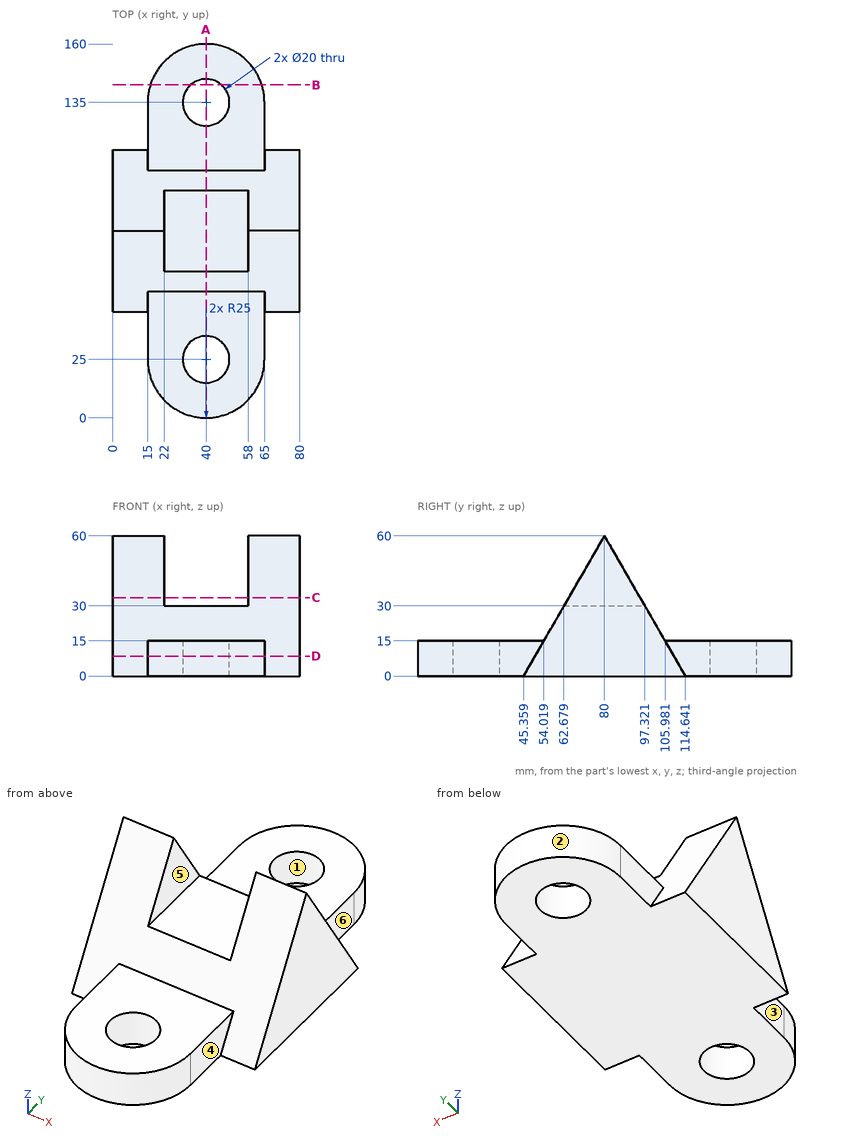
Study the drawing (mm; zero at the part's minimum x, y, z) and answer. A direction names the side the tool comes from. Round coordinates to 2 decimals unless told otherwise and drop trailing zeros. Write each loop counter-clockwise with the first axis right and the second up, starting at its lowest first coordinate (ties: lowest second). Pieces come first, ordered by that corner, then holes. Notation, with made-up numbers: (77.5, -40) - (110.5, -40) arc R13 cw to (110.5, -21) - close; hole circle Ø3 at (-10.5, 54.25). An arc over 180 degrees is marked (long way). Use a Markdown table: item, result. Add a question column.
1. For a pull along Y with two mould halves and no side action, classify the marked faces 1, 2 and 3 as +Y half, -Y half, draft (parallel to the pull), parting line (faces both ways), or undercut.
2. The part is cut by section C-C (z = 33.5). Write down the section's boundary in (x, y).
3. Consider line 1 (Y direction, x = 40, z = 5.5); line 2 (Z direction, x = 59, y = 121.5); line 3 (X direction, y = 126, z = 11) (1 decimal). Determine where each line is inside the solid, lowest interval first.
4. Flat-ended cylindrical pins translate along their axes: P1, Ø4.5, axis at y = 41, z = 5.5, coming from the -X side; P2, Ø6, axis at x = 57, z = 18.5, coming from the +Y side; P3, Ø1.5, axis at x = 26, z = 24, coming from the -Y side. Find the tip coordinate at first contact, or state that the pin passes through.
5. The part is cut by section B-B (y = 142.5). Write down the section's boundary in (x, z) (1 decimal), and give its area (3 significant figures).
6. The part is cut by section D-D (z = 8.5). Write down the section's boundary in (x, y), and give its area (3 significant figures).
7. The part is cut by section A-A (x = 40). Write down the section's boundary in (y, z).
8. A tool of negligible diameter and unlimited length cuts with its end or side. For the marked faces 4, 5 and 6, from which of +Z, -Z, +X, -X, +Y, -Y can it reach the whole face along a straight path? Write none if from no direction.
Reported:
| question | item | result |
|---|---|---|
| 1 | face 1 | undercut |
| 1 | face 2 | +Y half |
| 1 | face 3 | draft |
| 2 | outline | (0, 64.7) - (22, 64.7) - (22, 95.3) - (0, 95.3) - close; (58, 64.7) - (80, 64.7) - (80, 95.3) - (58, 95.3) - close |
| 3 | line 1 | 0 to 15, 35 to 125, 145 to 160 |
| 3 | line 2 | 0 to 15 |
| 3 | line 3 | 15 to 35.6, 44.4 to 65 |
| 4 | P1 | x = 15 |
| 4 | P2 | y = 105.69 |
| 4 | P3 | y = 58.78 |
| 5 | outline | (16.2, 0) - (33.4, 0) - (33.4, 15) - (16.2, 15) - close; (46.6, 0) - (63.8, 0) - (63.8, 15) - (46.6, 15) - close |
| 5 | area | 517 mm^2 |
| 6 | outline | (0, 50.27) - (15, 50.27) - (15, 25) arc R25 ccw to (65, 25) - (65, 50.27) - (80, 50.27) - (80, 109.73) - (65, 109.73) - (65, 135) arc R25 ccw to (15, 135) - (15, 109.73) - (0, 109.73) - close; hole circle Ø20 at (40, 25); hole circle Ø20 at (40, 135) |
| 6 | area | 8,620 mm^2 |
| 7 | outline | (0, 0) - (15, 0) - (15, 15) - (0, 15) - close; (35, 0) - (125, 0) - (125, 15) - (105.98, 15) - (97.32, 30) - (62.68, 30) - (54.02, 15) - (35, 15) - close; (145, 0) - (160, 0) - (160, 15) - (145, 15) - close |
| 8 | face 4 | +Z, +X, -Y |
| 8 | face 5 | +Z, +Y, -Y |
| 8 | face 6 | +Z, +X, +Y |
